Can you work these out from the model? Positions are in its coordinate system, mm. A direction names the side the tool comes from. Coordinates: 2 decimals unless noted, no trailing zeros. Order: outer loops, then holes, each group sorted by start corner. A loop starts at its lowest first (then second) coordinate and runs counter-clockwise, first axis right, second up.
```python
from build123d import *

# Parameters (mm, degrees)
BOSS_EXTRUDE1_DEPTH = 12
SKETCH2_R           = 0.8
CUT_EXTRUDE1_DEPTH  = 20


with BuildPart() as part:
    # Sketch1 → Boss-Extrude1 (new body)
    with BuildSketch(Plane.XY):
        with BuildLine():
            Line((-2.2, 0), (-2.2, -2.2))
            Line((-2.2, -2.2), (-6.5, -2.2))
            Line((-6.5, -2.2), (-6.5, 0))
            Line((-6.5, 0), (-3.4, 0))
            ThreePointArc((-3.4, 0), (0, 3.4), (3.4, 0))
            Line((3.4, 0), (6.5, 0))
            Line((6.5, 0), (6.5, -2.2))
            Line((6.5, -2.2), (2.2, -2.2))
            Line((2.2, -2.2), (2.2, 0))
            ThreePointArc((2.2, 0), (0, 2.2), (-2.2, 0))
        make_face()
    extrude(amount=BOSS_EXTRUDE1_DEPTH)

    # Sketch2 → Cut-Extrude1 (cut)
    with BuildSketch(Plane(origin=(0, 0, 0), x_dir=(1, 0, 0), z_dir=(0, 1, 0))):
        with Locations(Location((-4.95, -3, 0), (0, 0, 270))):
            Circle(SKETCH2_R)
        with Locations(Location((-4.95, -9, 0), (0, 0, 180))):
            Circle(SKETCH2_R)
        with Locations(Location((4.95, -3, 0), (0, 0, 180))):
            Circle(SKETCH2_R)
        with Locations(Location((4.95, -9, 0), (0, 0, 270))):
            Circle(SKETCH2_R)
    extrude(amount=-CUT_EXTRUDE1_DEPTH, mode=Mode.SUBTRACT)


solid = part.part
```
1. On a 3-axis mill with a long thin cutter (end or side, diameter ignored), from which of +Z, -Z, +X, -X, +Y, -Y can I reach the whole of each face in a straight line? I mean faces 5 (the flat face through (-5, 0, 6)), 6 (the flat face through (5, 0, 6)), 7 (the flat face through (2.2, -1, 6)). Say none if no direction works.
Completed:
face 5: +Z, -Z, -X, +Y
face 6: +Z, -Z, +X, +Y
face 7: +Z, -Z, -Y
2. I'm going to push flat-ended pins straight in: pin 1 (2.5 mm diameter, centred on x = 4.95, z = 3, fed in from +Y); pin 2 (1.3 mm diameter, centred on x = 4.95, z = 9, fed in from -Y); pin 3 (3.5 mm diameter, centred on x = 4.5, z = 8.5, fed in from +Y). Where does each tip first touch, or does it pass through?
Completed:
pin 1: stops at y = 0
pin 2: passes through
pin 3: stops at y = 2
3. Imagine slicing it at D-D on z = 1.5. Please give me the cut outline in (x, y).
Completed:
outline: (-6.5, -2.2) - (-2.2, -2.2) - (-2.2, 0) arc R2.2 cw to (2.2, 0) - (2.2, -2.2) - (6.5, -2.2) - (6.5, 0) - (3.4, 0) arc R3.4 ccw to (-3.4, 0) - (-6.5, 0) - close
4. Imagine slicing it at B-B on z = 3. Please give me the cut outline in (x, y).
Completed:
outline: (-6.5, -2.2) - (-5.75, -2.2) - (-5.75, 0) - (-6.5, 0) - close; (-4.15, -2.2) - (-2.2, -2.2) - (-2.2, 0) arc R2.2 cw to (2.2, 0) - (2.2, -2.2) - (4.15, -2.2) - (4.15, 0) - (3.4, 0) arc R3.4 ccw to (-3.4, 0) - (-4.15, 0) - close; (5.75, -2.2) - (6.5, -2.2) - (6.5, 0) - (5.75, 0) - close
5. Please list where these lines run through material, in increasing order: probe 1 along X at (y, z) = (-1.8, 11.5); probe 2 along Z at (x, y) = (-5.25, -1); probe 3 along Y at (x, z) = (-5.25, 1).
Completed:
probe 1: x = -6.5 to -2.2, 2.2 to 6.5
probe 2: z = 0 to 2.26, 3.74 to 8.26, 9.74 to 12
probe 3: y = -2.2 to 0
6. Thinking about a two-plate mould opening in X: for faces 1 (the cylindrical face through (5.58, -1.08, 2.51)), 2 (the flat face through (4, -2.2, 6)), 3 (the cylindrical face through (0, 2.2, 5.9)), 4 (the flat face through (6.5, -1, 6)), which applies, pulls with the +X half, pulls with the -X half, needs draft (parallel to the pull), parting line crosses it, or undercut?
Completed:
face 1: undercut
face 2: needs draft
face 3: undercut
face 4: pulls with the +X half
7. Imagine slicing it at C-C on x = -4.95. Please give me the cut outline in (y, z).
Completed:
outline: (-2.2, 0) - (0, 0) - (0, 2.2) - (-2.2, 2.2) - close; (-2.2, 3.8) - (0, 3.8) - (0, 8.2) - (-2.2, 8.2) - close; (-2.2, 9.8) - (0, 9.8) - (0, 12) - (-2.2, 12) - close
8. Imagine slicing it at A-A on y = -0.9. Please give me the cut outline in (x, z).
Completed:
outline: (-6.5, 0) - (-2.2, 0) - (-2.2, 12) - (-6.5, 12) - close; (2.2, 0) - (6.5, 0) - (6.5, 12) - (2.2, 12) - close; hole circle Ø1.6 at (-4.95, 3); hole circle Ø1.6 at (-4.95, 9); hole circle Ø1.6 at (4.95, 3); hole circle Ø1.6 at (4.95, 9)
